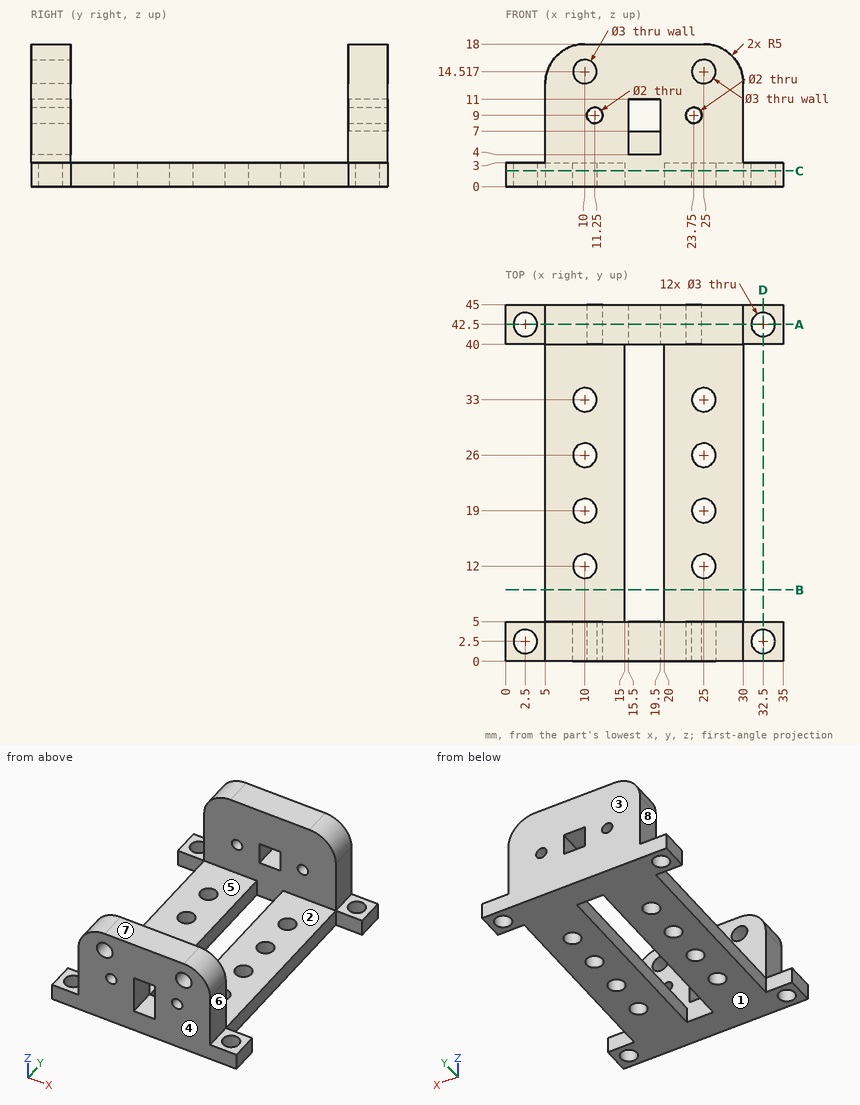
Here's the drawing with two shaded views (mm, measured from the low corner). I have some questions. A direction names the side the tool comes from. Coordinates: 2 decimals unless noted, no trailing zeros. Order: outer loops, then holes, each group sorted by start corner. A loop starts at its lowest first (then second) coordinate and runs counter-clockwise, first axis right, second up.
Q1. Will these pins go through, and if not, where does the flat tip stop? pin 1 (0.9 mm diameter, centred on y = 23, z = 1.5, fed in from +X); pin 2 (2.5 mm diameter, centred on y = 3, z = 8, fed in from -X); pin 3 (2 mm diameter, centred on x = 19.5, y = 8, fed in from +Z); pin 4 (1 mm diameter, centred on x = 31.5, y = 12.5, fed in from -Z).
Q2. Suppose I cut it at B-B on y = 9. Please give me the cut outline in (x, z).
Q3. Which directions (+Z, -Z, +X, -X, +Y, -Y) give clear straight access to the entire face, cutting with the end or side of a thin tool? Please do the marked faces 5, 6, 7 and 8.
Q4. Please list where these lines run through material, in increasing order: L1, parallel to Y at x = 25, z = 1.35; L2, parallel to Y at x = 24, z = 6.5; L3, parallel to Y at x = 2.5, z = 1.45.
Q5. Suppose I cut it at C-C on z = 2. Give the number of separate pieces and of enclosed holes in the cut face, and give its area (3 significant figures).
Q6. Thinking about a two-plate mould opening in Y: for the marked faces 1, 2, 3 and 4, which applies, released by +Y, released by -Y, zero draft, split by the parting line, or undercut?
Q7. Suppose I cut it at A-A on y = 42.5. Please give me the cut outline in (x, z), and give its area (3 significant figures).
Q8. Suppose I cut it at D-D on x = 32.5. Please give me the cut outline in (y, z), and give its area (3 significant figures).
Answer:
1. pin 1: stops at x = 30
1. pin 2: stops at x = 5
1. pin 3: stops at z = 3
1. pin 4: passes through
2. outline: (5, 0) - (15, 0) - (15, 3) - (5, 3) - close; (20, 0) - (30, 0) - (30, 3) - (20, 3) - close
3. face 5: +Z, +X, -X
3. face 6: +Z, +X, +Y, -Y
3. face 7: +Z, +X, -X, +Y, -Y
3. face 8: +Z, -X, +Y, -Y
4. L1: y = 0 to 10.5, 13.5 to 17.5, 20.5 to 24.5, 27.5 to 31.5, 34.5 to 45
4. L2: y = 0 to 5, 40 to 45
4. L3: y = 0 to 1, 4 to 5, 40 to 41, 44 to 45
5. separate pieces: 1
5. enclosed holes: 13
5. area: 965 mm2
6. face 1: zero draft
6. face 2: undercut
6. face 3: released by +Y
6. face 4: released by -Y
7. outline: (0, 0) - (1, 0) - (1, 3) - (0, 3) - close; (4, 0) - (31, 0) - (31, 3) - (30, 3) - (30, 13) arc R5 ccw to (25, 18) - (10, 18) arc R5 ccw to (5, 13) - (5, 3) - (4, 3) - close; (34, 0) - (35, 0) - (35, 3) - (34, 3) - close; hole circle Ø2 at (11.25, 9); hole (15.5, 7) - (19.5, 7) - (19.5, 11) - (15.5, 11) - close; hole circle Ø2 at (23.75, 9)
7. area: 429 mm2
8. outline: (0, 0) - (1, 0) - (1, 3) - (0, 3) - close; (4, 0) - (5, 0) - (5, 3) - (4, 3) - close; (40, 0) - (41, 0) - (41, 3) - (40, 3) - close; (44, 0) - (45, 0) - (45, 3) - (44, 3) - close
8. area: 12.0 mm2
